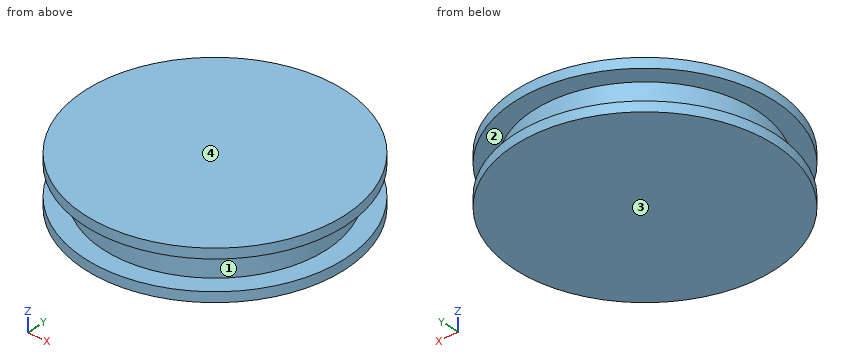
from build123d import *

# Parameters (mm, degrees)
F2_R     = 52.5
F3_DEPTH = 4
F5_R     = 45
F6_DEPTH = 12
F8_R     = 52.5
F9_DEPTH = 4


with BuildPart() as f3:
    # F2 (on Top) → F3 (new body)
    with BuildSketch(Plane.XY):
        Circle(F2_R)
    extrude(amount=F3_DEPTH)

    # F5 (on offset) → F6 (join)
    with BuildSketch(Plane.XY.offset(4)):
        Circle(F5_R)
    extrude(amount=F6_DEPTH)

    # F8 (on offset) → F9 (join)
    with BuildSketch(Plane.XY.offset(16)):
        Circle(F8_R)
    extrude(amount=F9_DEPTH)


with BuildPart() as f10_1:
    # F10: copy of F3
    add(f3.part.moved(Location((0, 0, 20))))


with BuildPart() as f12_1:
    # F12: copy of F3
    add(f3.part)


with BuildPart() as f3_1:
    # F14: moved
    add(f3.part.moved(Location((0, 0, 20))))


solid = f3_1.part
Build history of the part. All positions in model axes, mm. Face numbers are marked on the shaded views. Coordinates: 2 decimals unless noted, no trailing zeros. Order: outer loops, then holes, each group sorted by start corner. A loop starts at its lowest first (then second) coordinate and runs counter-clockwise, first axis right, second up. Notation, with made-up numbers: (-33, -2) - (19, -2) arc R14 cw to (19, 23) - close; hole circle Ø2 at (6.5, -18.5). An arc over 180 degrees is marked (long way). Write item = value, one per line. Start each with the question number.
1) Flat gauge pins, fed straight in: pin 1 Ø1.5 at (x, z) = (-40.5, 29.5) entering from +Y; pin 2 Ø12 at (y, z) = (16, 35) entering from +X; pin 3 Ø1.5 at (x, z) = (24.5, 34.5) entering from +Y. Where does each tip first touch, or does it go through?
2) Wall check: line 1 along Z through (x, y) = (36.5, -29.5); line 2 along X through (y, z) = (27, 38.5) (3 decimals); line 3 along X through (y, z) = (-12, 23). Give the ranges that are in metal, low to high. Write a range as from..to.
3) Two-plate mould, pull along Z, no slides. Class the marked faces 1, 2, 3 and 4: pulls with the +Z half, pulls with the -Z half, needs draft (parallel to the pull), parting line crosses it, or undercut.
4) Saw through at C-C on z = 22. Write the cut outline in (x, y).
5) Saw through at A-A on y = 0. Write the cut outline in (x, z), then the cut area to 3 significant figures.
6) Saw through at D-D on z = 31.5. Write the cut outline in (x, y), then the cut area to 3 significant figures.
From the geometry:
q1.pin_1 = 21.09
q1.pin_2 = 51.52
q1.pin_3 = 38.22
q2.line_1 = 20..24, 36..40
q2.line_2 = -45.025..45.025
q2.line_3 = -51.11..51.11
q3.face_1 = undercut
q3.face_2 = undercut
q3.face_3 = pulls with the -Z half
q3.face_4 = pulls with the +Z half
q4.outline = circle Ø105 at (0, 0)
q5.outline = (-52.5, 20) - (52.5, 20) - (52.5, 24) - (45, 24) - (45, 36) - (52.5, 36) - (52.5, 40) - (-52.5, 40) - (-52.5, 36) - (-45, 36) - (-45, 24) - (-52.5, 24) - close
q5.area = 1,920 mm^2
q6.outline = circle Ø90 at (0, 0)
q6.area = 6,360 mm^2
